Can you work these out from the model? Positions are in its coordinate system, mm. A direction names the side the tool comes from. Round coordinates to 2 decimals unless told otherwise and drop trailing zeros. Write item = value, one per line.
from build123d import *

# Parameters (mm, degrees)
SKETCH7_R          = 152.4
CUT_EXTRUDE1_DEPTH = 147.399141516
SKETCH17_R         = 4.7625
CUT_EXTRUDE4_DEPTH = 147.399141516
CIRPATTERN2_COUNT  = 6


with BuildPart() as part:
    # Sketch6 → Revolve1 (revolve)
    with BuildSketch(Plane.XY, mode=Mode.PRIVATE) as revolve1_sk:
        with BuildLine():
            Line((50.8, 22.53035676), (50.8, 6.35))
            Line((50.8, 6.35), (53.975, 6.35))
            Line((53.975, 6.35), (53.975, 20.227565916))
            add(Edge.make_bspline(
                [(53.975, 20.227565916), (54.291634879, 20.330430839), (55.162475518, 20.612719168), (56.636149311, 21.087725347), (58.867170376, 21.80102074), (61.522421046, 22.638682883), (64.736507837, 23.637812157), (68.023541536, 24.646609183), (72.39438926, 25.969741612), (77.802325895, 27.573199633), (84.37229967, 29.477097548), (93.118193973, 31.954107645), (108.466778526, 36.165197289), (130.491628823, 41.875745108), (165.870302673, 50.489926314), (210.303076361, 60.449379541), (281.693068548, 75.067985253), (371.347473816, 91.310304544), (479.374979471, 108.229836311), (569.684892552, 120.376775068), (642.076792345, 128.912483065), (696.438363769, 134.692640498), (750.863527692, 139.800693107), (796.267539796, 143.42521879), (832.617797313, 145.860290015), (859.890749047, 147.416222506), (882.628689993, 148.436275801), (898.53412358, 148.946546098), (907.62769622, 149.150954449), (912.14731785, 149.217348506), (914.4107585, 149.225018228)],
                knots=[0.06148136, 0.06148136, 0.06148136, 0.06148136, 0.06256458, 0.064402689, 0.066240798, 0.069917015, 0.073593232, 0.07726945, 0.080945667, 0.088298102, 0.095650536, 0.103002971, 0.11770784, 0.147117579, 0.176527318, 0.235346795, 0.294166272, 0.411805227, 0.529444182, 0.647083136, 0.705902613, 0.764722091, 0.823541568, 0.882361045, 0.911770784, 0.941180523, 0.970590261, 0.985295131, 0.992647565, 1, 1, 1, 1], degree=3))
            Line((914.4107585, 149.225018228), (914.4107585, 146.05))
            Line((914.4107585, 146.05), (1066.8, 146.05))
            Line((1066.8, 146.05), (1066.8, 149.225))
            Line((1066.8, 149.225), (965.2, 149.225))
            Line((965.2, 149.225), (965.2, 152.4))
            Line((965.2, 152.4), (914.4, 152.4))
            add(Edge.make_bspline(
                [(50.8, 22.53035676), (51.62596102, 22.801930188), (53.247366667, 23.331443773), (57.113810342, 24.581671091), (62.137627853, 26.163245596), (68.472923462, 28.113411094), (76.389796689, 30.474842786), (85.386033894, 33.081102875), (95.241355255, 35.841520364), (106.104903016, 38.788706559), (117.812200959, 41.867831442), (130.423899043, 45.08497442), (143.907449646, 48.417167108), (158.285989872, 51.860839853), (172.682057827, 55.208017205), (187.101006341, 58.468808185), (201.536340401, 61.648015415), (215.98908439, 64.751824582), (234.073297096, 68.542392147), (255.802551989, 72.956576003), (281.189453131, 77.92470015), (306.614812158, 82.692611325), (328.432361696, 86.646151134), (350.268122203, 90.497714312), (372.121192631, 94.250003895), (397.640090518, 98.488121242), (426.834492226, 103.147632175), (456.056824987, 107.628600482), (485.305388678, 111.934967932), (514.578772116, 116.069226586), (543.875783343, 120.032588186), (573.19542697, 123.82488003), (602.536868801, 127.444739672), (631.89942018, 130.889153604), (661.282519219, 134.153873932), (698.036524214, 138.001817701), (742.180870702, 142.229994267), (786.373789985, 145.926990276), (830.615211008, 148.98950394), (864.145536025, 150.817451898), (884.93243709, 151.702539519), (900.347440379, 152.177178216), (908.376949057, 152.340862845), (912.39222778, 152.393196617), (914.4, 152.4)],
                knots=[0.058888363, 0.058888363, 0.058888363, 0.058888363, 0.058888363, 0.06286181, 0.066835256, 0.074782149, 0.082729042, 0.090675935, 0.102752696, 0.114829458, 0.126906219, 0.138982981, 0.154876753, 0.170770526, 0.186664299, 0.202558071, 0.218451844, 0.234345618, 0.250239391, 0.266133165, 0.297920711, 0.329708258, 0.361495805, 0.377389579, 0.393283353, 0.4250709, 0.456858447, 0.488645994, 0.52043354, 0.552221087, 0.584008633, 0.615796181, 0.647583729, 0.679371276, 0.711158823, 0.74294637, 0.774733917, 0.838309011, 0.901884107, 0.933671654, 0.965459201, 0.9827296, 0.9913648, 1, 1, 1, 1, 1], degree=4))
        make_face()
    revolve(revolve1_sk.sketch.rotate(Axis((-61.64472501, 0, 0), (1, 0, 0)), 90), axis=Axis((-61.64472501, 0, 0), (1, 0, 0)))

    # Sketch7 → Cut-Extrude1 (cut)
    with BuildSketch(Plane(origin=(965.2, 0, 0), x_dir=(0, 0, -1), z_dir=(1, 0, 0))):
        with Locations(Location((0, 0, 0), (0, 0, 180))):
            Circle(SKETCH7_R)
    extrude(amount=CUT_EXTRUDE1_DEPTH, mode=Mode.SUBTRACT)

    # Sketch17 → Cut-Extrude4 (cut)
    with BuildSketch(Plane(origin=(0, 152.4, 0), x_dir=(1, 0, 0), z_dir=(0, 1, 0))):
        with Locations(Location((939.8, 0, 0), (0, 0, 270))):
            Circle(SKETCH17_R)
    cut_extrude4 = extrude(amount=-CUT_EXTRUDE4_DEPTH, mode=Mode.SUBTRACT)

    # CirPattern2: Cut-Extrude4 ×6 about axis
    cirpattern2_axis = Axis((0, 0, 0), (1, 0, 0))
    for i in range(1, CIRPATTERN2_COUNT):
        add(cut_extrude4.rotate(cirpattern2_axis, i * 360 / CIRPATTERN2_COUNT), mode=Mode.SUBTRACT)


solid = part.part
1. We'd pull the mould along Z, two halves only. Please class faces 4 (the flat face through (53.975, -5, 5)), 5 (the flat face through (965.2, 123.5, -78.3)), 6 (the cylindrical face through (939.444, 148.776, -33.037)): released by +Z, released by -Z, zero draft, split by the parting line, or undercut.
Entries:
face_4 = undercut
face_5 = zero draft
face_6 = split by the parting line
2. I need wall thicknesses on line 1 (Z direction, x = 902, y = 29); line 2 (Z direction, x = 798.5, y = 22); line 3 (Y direction, x = 787, z = -63). Which ranges of each line are inside material? Lowest first, please. Write a range as [from, to].
Entries:
line_1 = [-149.41, -146.17], [146.17, 149.41]
line_2 = [-145.02, -141.8], [141.8, 145.02]
line_3 = [-131.51, -127.97], [127.97, 131.51]
3. I'm going to push flat-ended pins straight in: pin 1 (1.5 mm diameter, centred on x = 207, y = -44, fed in from +Z); pin 2 (3 mm diameter, centred on x = 252, z = -63, fed in from -Y); pin 3 (12 mm diameter, centred on x = 863.5, y = 59, fed in from +Z). Where does each tip first touch, or does it pass through?
Entries:
pin_1 = 45.59
pin_2 = -37.81
pin_3 = 141.12
4. For faces 1 (the cylindrical face through (940.161, 129.571, 67.393)), 2 (the flat face through (50.8, 5, 5)), 3 (the flat face through (914.411, 110, 99)), which set-ups out of +Z, -Z, +X, -X, +Y, -Y let a thin tool reach every point of the face, with its end or its side?
Entries:
face_1 = +X
face_2 = +Z, -Z, -X, +Y, -Y
face_3 = none
